Design review of the part shown in the three views and the two pictorial views. Dimensions are in mm from the part's minimum x, y and z. Round coordinates to 2 decimals unless told otherwise and drop trailing zeros. Order: outer loops, then holes, each group sorted by start corner. A loop starts at its lowest first (then second) coordinate and runs counter-clockwise, first axis right, second up.
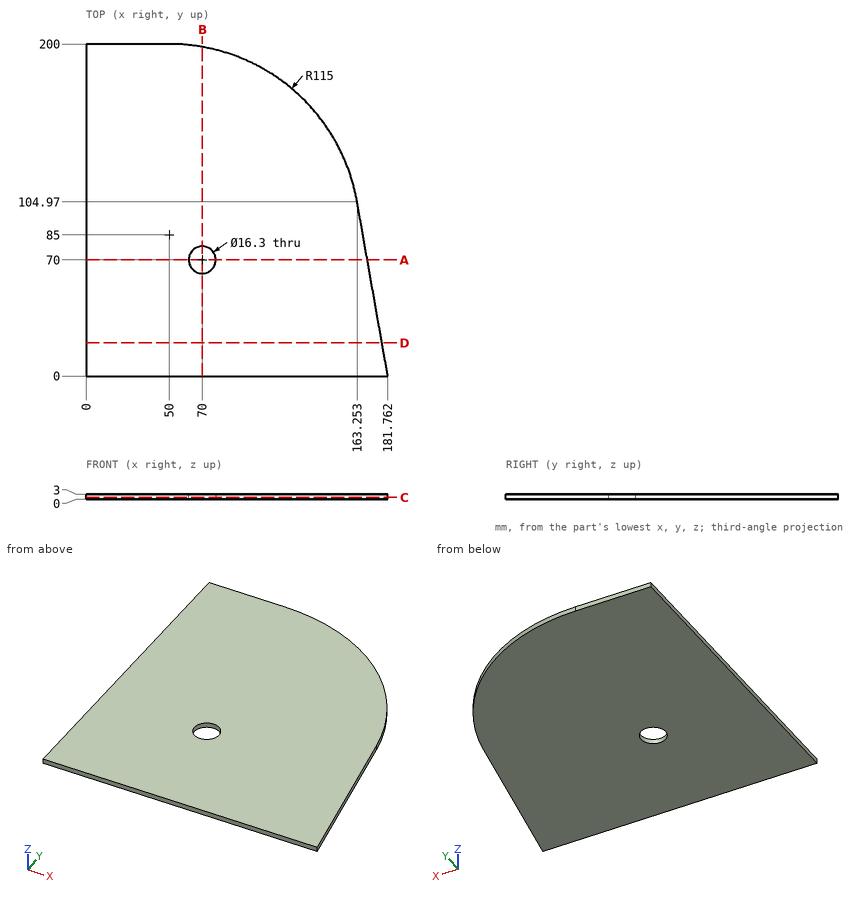
1) Take a section at B-B on x = 70. Give the boundary of the cut face in (y, z).
Results:
outline: (0, 0) - (61.85, 0) - (61.85, 3) - (0, 3) - close; (78.15, 0) - (198.25, 0) - (198.25, 3) - (78.15, 3) - close
2) Take a section at A-A on y = 70. Give the boundary of the cut face in (x, z).
Results:
outline: (0, 0) - (61.85, 0) - (61.85, 3) - (0, 3) - close; (78.15, 0) - (169.42, 0) - (169.42, 3) - (78.15, 3) - close
3) Take a section at C-C on z = 1.1. Give the boundary of the cut face in (x, y), plus the area to 3 significant figures.
Results:
outline: (0, 0) - (181.76, 0) - (163.25, 104.97) arc R115 ccw to (50, 200) - (0, 200) - close; hole circle Ø16.3 at (70, 70)
area: 30,800 mm2
4) Take a section at D-D on y = 20. Give the boundary of the cut face in (x, z) (1 decimal).
Results:
outline: (0, 0) - (178.2, 0) - (178.2, 3) - (0, 3) - close
5) To check wall thickness, follow line 1 along X through (y, z) = (186, 2.2) (1 decimal); line 2 along Y through (x, z) = (70, 1.5); line 3 along X through (y, z) = (151.5, 0.6) (1 decimal). State the ranges of each line that lie inside material, in increasing order.
Results:
line 1: x = 0 to 105
line 2: y = 0 to 61.85, 78.15 to 198.25
line 3: x = 0 to 143.8
